from build123d import *

# Parameters (mm, degrees)
SKETCH1_R           = 60.3504
SKETCH1_R_2         = 3.175
BOSS_EXTRUDE1_DEPTH = 6


with BuildPart() as part:
    # Sketch1 → Boss-Extrude1 (new body)
    with BuildSketch(Plane(origin=(0, 0, 0), x_dir=(1, 0, 0), z_dir=(0, 1, 0))):
        Circle(SKETCH1_R)
        Circle(SKETCH1_R_2, mode=Mode.SUBTRACT)
        with Locations((0, -54.0004)):
            Circle(SKETCH1_R_2, mode=Mode.SUBTRACT)
        with Locations((-46.765718215, 27.0002)):
            Circle(SKETCH1_R_2, mode=Mode.SUBTRACT)
        with Locations((46.765718215, 27.0002)):
            Circle(SKETCH1_R_2, mode=Mode.SUBTRACT)
    extrude(amount=BOSS_EXTRUDE1_DEPTH)


solid = part.part
Geometry check sheet. Reference: the model listing, model coordinates, mm. Round coordinates to 2 decimals unless told otherwise and drop trailing zeros. Order: outer loops, then holes, each group sorted by start corner. A loop starts at its lowest first (then second) coordinate and runs counter-clockwise, first axis right, second up. Notation, with made-up numbers: M 35.5,-24.75 L 48.5,-24.75 A17 cw 48.5,5.25 Z; hole C 50.25,82.5 d6. An arc over 180 degrees is marked long. Answer in a Markdown table with one row per item. Add a question column.
Item 1: Material ranges on L1, parallel to Z at x = 0, y = 3.25 (3 decimals); L2, parallel to Z at x = -49, y = 1.4; L3, parallel to Z at x = 45.5, y = 2.4, recorded low to high. Write a range as [from, to].
Item 2: Draft check along Z on faces 1 (the face through (13, 6, -1)), 2 (the face through (-0.69, 2.96, 3.1)), 3 (the face through (-47.892, 2.958, 36.722)), 4 (the face through (1.707, 2.958, 51.323)). Enter one of: released by +Z, released by -Z, zero draft, split by the parting line, or undercut.
Item 3: Sectioned sample at D-D, the plane x = -15. Enter the section's corners in (y, z), plus the area to 3 significant figures.
Item 4: Sectioned sample at A-A, the plane z = 0. Enter the section's corners in (x, y) (3 decimals), plus the area to 3 significant figures.
Item 5: Depth check by flat-ended pin: pin 1 Ø1 at (x, y) = (6, 2) entering from +Z; pin 2 Ø1.5 at (x, y) = (7, 4) entering from +Z; pin 3 Ø5.5 at (x, z) = (46.77, -27) entering from +Y; pin 4 Ø3 at (y, z) = (2.5, -40.5) entering from -X. Enter the tip coordinate at first touch or a pass-through.
Item 6: Sectioned sample at C-C, the plane y = 1.05. Enter the section's corners in (x, z) (3 decimals), plus the area to 3 significant figures.
Item 7: Sectioned sample at B-B, the plane x = 0. Enter the section's corners in (y, z) (3 decimals).
Filled in:
| question | item | result |
|---|---|---|
| 1 | L1 | z = [-60.35, -3.175], [3.175, 50.825], [57.175, 60.35] |
| 1 | L2 | z = [-35.23, -29.26], [-24.74, 35.23] |
| 1 | L3 | z = [-39.65, -29.91], [-24.09, 39.65] |
| 2 | face 1 | zero draft |
| 2 | face 2 | undercut |
| 2 | face 3 | split by the parting line |
| 2 | face 4 | undercut |
| 3 | outline | M 0,-58.46 L 6,-58.46 L 6,58.46 L 0,58.46 Z |
| 3 | area | 701 mm² |
| 4 | outline | M -60.35,0 L -3.175,0 L -3.175,6 L -60.35,6 Z; M 3.175,0 L 60.35,0 L 60.35,6 L 3.175,6 Z |
| 4 | area | 686 mm² |
| 5 | pin 1 | stops at z = 60.1 |
| 5 | pin 2 | stops at z = 60.03 |
| 5 | pin 3 | passes through |
| 5 | pin 4 | stops at x = -46.06 |
| 6 | outline | C 0,0 d120.701; hole C -46.766,-27 d6.35; hole C 0,0 d6.35; hole C 0,54 d6.35; hole C 46.766,-27 d6.35 |
| 6 | area | 11,300 mm² |
| 7 | outline | M 0,-60.35 L 6,-60.35 L 6,-3.175 L 0,-3.175 Z; M 0,3.175 L 6,3.175 L 6,50.825 L 0,50.825 Z; M 0,57.175 L 6,57.175 L 6,60.35 L 0,60.35 Z |
